```python
from build123d import *

# Parameters (mm, degrees)
SKETCH1_R           = 3.556
BOSS_EXTRUDE1_DEPTH = 83.53298
FILLET1_R           = 3.556


with BuildPart() as part:
    # Sketch1 → Boss-Extrude1 (new body)
    with BuildSketch(Plane(origin=(0, 0, 0), x_dir=(1, 0, 0), z_dir=(0, 1, 0))):
        with Locations(Location((0, 0, 0), (0, 0, 270))):
            Circle(SKETCH1_R)
    extrude(amount=BOSS_EXTRUDE1_DEPTH)

    # Sketch2 → Cut-Revolve2 (revolve, cut)
    with BuildSketch(Plane(origin=(0, 100.014806598, -21.087436426), x_dir=(0, -1, 0), z_dir=(1, 0, 0))):
        with BuildLine():
            Line((90.695546598, -17.531436426), (87.520546598, -17.531436426))
            Line((87.520546598, -17.531436426), (88.478687606, -18.489577434))
            ThreePointArc((88.478687606, -18.489577434), (88.736198639, -18.661640805), (89.039953613, -18.722061426))
            Line((89.039953613, -18.722061426), (89.901796598, -18.722061426))
            ThreePointArc((89.901796598, -18.722061426), (90.463062606, -18.489577434), (90.695546598, -17.928311426))
            Line((90.695546598, -17.928311426), (90.695546598, -17.531436426))
        make_face()
    revolve(axis=Axis((0, 0, 0), (0, 1, 0)), mode=Mode.SUBTRACT)

    # Fillet1
    fillet1_edges = [part.edges().sort_by_distance(p)[0] for p in [
        (0, 0, -3.556),
    ]]
    fillet(fillet1_edges, radius=FILLET1_R)


solid = part.part
```
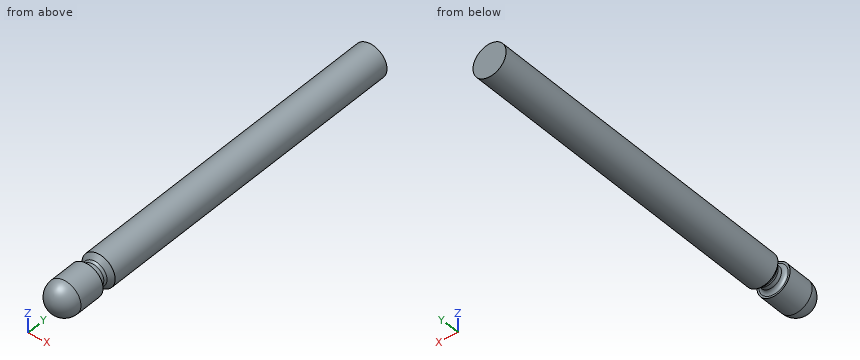
CAD build for the part. Positions are in the model's coordinates, mm. Coordinates: 2 decimals unless noted, no trailing zeros. Write each loop counter-clockwise with the first axis right and the second up, starting at its lowest first coordinate (ties: lowest second). Pieces come first, ordered by that corner, then holes. Notation, with made-up numbers: (-11.5, 17) -> (42.5, 17) arc R16 cw to (42.5, 44) -> close; hole circle Ø2 at (8.25, -37.75). An arc over 180 degrees is marked (long way). Use CSV: the item, a comma, the result in double quotes. Start each with the question number.
Item 1: Band-saw the part on B-B, the plane x = 0. Write the cut outline in (y, z).
Item 2: Band-saw the part on C-C, the plane y = 42. Write the cut outline in (x, z).
Item 3: Wall check: probe 1 along Y at (x, z) = (-2.25, 2); probe 2 along Y at (x, z) = (2.5, 2); probe 3 along X at (y, z) = (73, 1.5). Give the ranges that are in metal, low to high.
Item 4: Band-saw the part on A-A, the plane z = 0. Write the cut outline in (x, y).
Item 5: Drop flat-ended pins along their axis: P1, Ø3, axis at y = 65.5, z = -2.5, coming from the +X side; P2, Ø2, axis at y = 60.5, z = 2, coming from the -X side. Give the stop position or say it passes through.
Response values:
1,outline,"(3.56, -3.56) -> (9.32, -3.56) -> (9.32, -3.16) arc R0.79 cw to (10.11, -2.37) -> (10.97, -2.37) arc R0.79 cw to (11.54, -2.6) -> (12.49, -3.56) -> (83.53, -3.56) -> (83.53, 3.56) -> (12.49, 3.56) -> (11.54, 2.6) arc R0.79 cw to (10.97, 2.37) -> (10.11, 2.37) arc R0.79 cw to (9.32, 3.16) -> (9.32, 3.56) -> (3.56, 3.56) arc R3.56 ccw to start"
2,outline,"circle Ø7.11 at (0, 0)"
3,probe 1,"y = 1.66 to 9.33, 11.95 to 83.53"
3,probe 2,"y = 2.01 to 9.32, 12.14 to 83.53"
3,probe 3,"x = -3.22 to 3.22"
4,outline,"(-3.56, 3.56) arc R3.56 ccw to (3.56, 3.56) -> (3.56, 9.32) -> (3.16, 9.32) arc R0.79 cw to (2.37, 10.11) -> (2.37, 10.97) arc R0.79 cw to (2.6, 11.54) -> (3.56, 12.49) -> (3.56, 83.53) -> (-3.56, 83.53) -> (-3.56, 12.49) -> (-2.6, 11.54) arc R0.79 cw to (-2.37, 10.97) -> (-2.37, 10.11) arc R0.79 cw to (-3.16, 9.32) -> (-3.56, 9.32) -> close"
5,P1,"stops at x = 3.41"
5,P2,"stops at x = -3.41"
